Verification items for the finished model (mm, model axes). Face numbers are marked on the shaded views. A direction names the side the tool comes from. Coordinates: 2 decimals unless noted, no trailing zeros. Loops run counter-clockwise (first coordinate to the right, second up) from the corner with the lowest first, then second, coordinate; pieces in that order, holes last. Notation, with made-up numbers: (-20.5, -29) -> (28.5, -29) arc R34 cw to (28.5, 7) -> close; hole circle Ø3 at (42, -19.75). An arc over 180 degrees is marked (long way). Write item = value, one per line.
```python
from build123d import *

# Parameters (mm, degrees)
SKETCH2_R           = 112.5
BOSS_EXTRUDE1_DEPTH = 28
SKETCH4_R           = 60
BOSS_EXTRUDE5_DEPTH = 50
FILLET2_R           = 3
FILLET3_R           = 10
SKETCH7_R           = 32.5
BOSS_EXTRUDE7_DEPTH = 100
SKETCH8_R           = 27.5
CUT_EXTRUDE1_DEPTH  = 239.73939767
SKETCH9_R           = 10
CUT_EXTRUDE2_DEPTH  = 219.660696057
FILLET4_R           = 5


with BuildPart() as part:
    # Sketch2 → Boss-Extrude1 (new body)
    with BuildSketch(Plane.XY):
        Circle(SKETCH2_R)
    extrude(amount=BOSS_EXTRUDE1_DEPTH)

    # Sketch4 → Boss-Extrude5 (add)
    with BuildSketch(Plane.XY.offset(28)):
        Circle(SKETCH4_R)
    extrude(amount=BOSS_EXTRUDE5_DEPTH)

    # Fillet2
    fillet2_edges = [part.edges().sort_by_distance(p)[0] for p in [
        (-60, 0, 28),
    ]]
    fillet(fillet2_edges, radius=FILLET2_R)

    # Fillet3
    fillet3_edges = [part.edges().sort_by_distance(p)[0] for p in [
        (-60, 0, 78),
    ]]
    fillet(fillet3_edges, radius=FILLET3_R)

    # Sketch7 → Boss-Extrude7 (add)
    with BuildSketch(Plane.XY.offset(78)):
        Circle(SKETCH7_R)
    extrude(amount=BOSS_EXTRUDE7_DEPTH)

    # Sketch8 → Cut-Extrude1 (cut, through all)
    with BuildSketch(Plane.XY.offset(178)):
        Circle(SKETCH8_R)
    extrude(amount=-CUT_EXTRUDE1_DEPTH, mode=Mode.SUBTRACT)

    # Sketch9 → Cut-Extrude2 (cut, through all)
    with BuildSketch(Plane.XY.offset(28)):
        with Locations((0, 86.25)):
            Circle(SKETCH9_R)
        with Locations((86.25, 0)):
            Circle(SKETCH9_R)
        with Locations((0, -86.25)):
            Circle(SKETCH9_R)
        with Locations((-86.25, 0)):
            Circle(SKETCH9_R)
    extrude(amount=-CUT_EXTRUDE2_DEPTH, mode=Mode.SUBTRACT)

    # Fillet4
    fillet4_edges = [part.edges().sort_by_distance(p)[0] for p in [
        (-32.5, 0, 178),
    ]]
    fillet(fillet4_edges, radius=FILLET4_R - 0.0001)  # a hair under: the kernel refuses the full size


solid = part.part
```
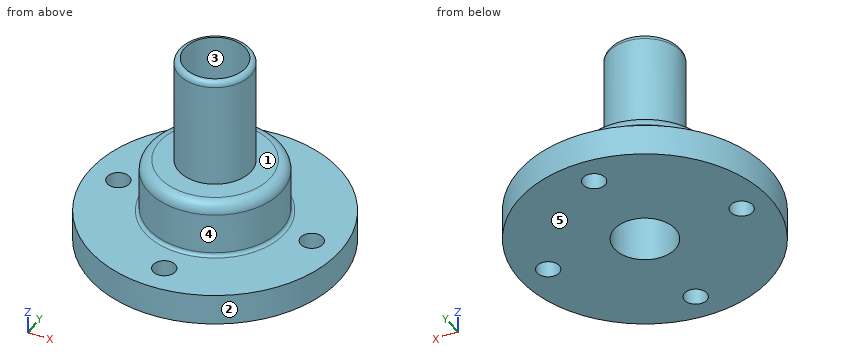
1) Sectioned sample at D-D, the plane x = 86.25. Record the cut outline in (y, z), plus the area to 3 significant figures.
Ans:
outline = (-72.23, 0) -> (-10, 0) -> (-10, 28) -> (-72.23, 28) -> close; (10, 0) -> (72.23, 0) -> (72.23, 28) -> (10, 28) -> close
area = 3,480 mm2
2) Release check for a two-part mould opening along Y. For the marked faces 3, 4 and 5 record: pulls with the +Y half, pulls with the -Y half, needs draft (parallel to the pull), parting line crosses it, or undercut.
Ans:
face_3 = undercut
face_4 = parting line crosses it
face_5 = needs draft
3) Tool access check on the marked faces 1 and 2. Record the directions out of +Z, -Z, +X, -X, +Y, -Y that give a thin tool (end or side, any length) a straight path to the whole face; none if there is none.
Ans:
face_1 = +Z
face_2 = +Z, -Z
4) Sectioned sample at A-A, the plane x = 0. Count the separate pieces of the cut face and the enclosed holes in it, plus the area to 3 significant figures.
Ans:
separate_pieces = 4
enclosed_holes = 0
area = 7,840 mm2
5) Depth check by flat-ended pin: pin 1 Ø10 at (x, y) = (89.5, 5.5) entering from +Z; pin 2 Ø1 at (y, z) = (-19, 93.5) entering from +X; pin 3 Ø10 at (x, z) = (24.5, 80) entering from -Y. Enter the tip coordinate at first touch or a pass-through.
Ans:
pin_1 = 28
pin_2 = 26.72
pin_3 = -52.06
6) Sectioned sample at C-C, the plane z = 105. Record the cut outline in (x, y).
Ans:
outline = circle Ø65 at (0, 0); hole circle Ø55 at (0, 0)
7) Material ranges on line 1 (Y direction, x = 0, z = 136); line 2 (Y direction, x = 0, z = 6.25); line 3 (Y direction, x = -2, z = 160.5), recorded low to high.
Ans:
line_1 = -32.5 to -27.5, 27.5 to 32.5
line_2 = -112.5 to -96.25, -76.25 to -27.5, 27.5 to 76.25, 96.25 to 112.5
line_3 = -32.44 to -27.43, 27.43 to 32.44
